Build history of the part. All positions in model axes, mm. Face numbers are marked on the shaded views. A direction names the side the tool comes from. Coordinates: 2 decimals unless noted, no trailing zeros. Loops run counter-clockwise (first coordinate to the right, second up) from the corner with the lowest first, then second, coordinate; pieces in that order, holes last. Notation, with made-up numbers: (81, -2.5) - (93, -2.5) arc R21 ccw to (93, 18.5) - close; hole circle Ø4 at (43.25, 16). An arc over 180 degrees is marked (long way). One line per item, written item: value.
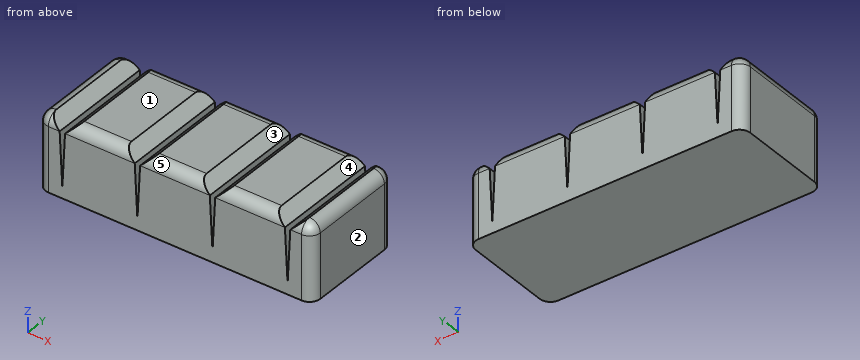
```python
from build123d import *

# Parameters (mm, degrees)
F1_DEPTH = 50
F2_SIZE  = 5
F3_R     = 4.99999


# Not quite as in the source:
# - a fillet or chamfer is up to 0.001 mm smaller than in the source, because OpenCascade refuses the exact size


with BuildPart() as f1:
    # F0 (on Front) → F1 (new body)
    with BuildSketch(Plane.XZ):
        Polygon((-62.637026581, 14.7639395539), (-62.637026581, -20.2360604461), (65.362973419, -20.2360604461), (65.362973419, 14.7639395539), (55.362973419, 14.7639395539), (53.862973419, -15.2360604461), (52.362973419, 14.7639395539), (20.362973419, 14.7639395539), (18.862973419, -15.2360604461), (17.362973419, 14.7639395539), (-14.637026581, 14.7639395539), (-16.137026581, -15.2360604461), (-17.637026581, 14.7639395539), (-49.637026581, 14.7639395539), (-51.137026581, -15.2360604461), (-52.637026581, 14.7639395539), align=None)
    extrude(amount=F1_DEPTH)

    # F2
    f2_edges = [f1.edges().sort_by_distance(p)[0] for p in [
        (-52.637027, -25, 14.76394),
        (-49.637027, -25, 14.76394),
        (-17.637027, -25, 14.76394),
        (-14.637027, -25, 14.76394),
        (17.362973, -25, 14.76394),
        (20.362973, -25, 14.76394),
        (52.362973, -25, 14.76394),
        (55.362973, -25, 14.76394),
    ]]
    chamfer(f2_edges, length=F2_SIZE)

    # F3 (radius 5 in the source; OpenCascade refuses exactly that, so slightly less here)
    f3_edges = [f1.edges().sort_by_distance(p)[0] for p in [
        (-62.637027, -25, 14.76394),
        (-60.137027, -50, 14.76394),
        (-60.137027, 0, 14.76394),
        (-33.637027, -50, 14.76394),
        (-33.637027, 0, 14.76394),
        (1.362973, 0, 14.76394),
        (1.362973, -50, 14.76394),
        (36.362973, -50, 14.76394),
        (36.362973, 0, 14.76394),
        (62.862973, -50, 14.76394),
        (65.362973, -25, 14.76394),
        (62.862973, 0, 14.76394),
        (-62.637027, -50, -2.73606),
        (-62.637027, 0, -2.73606),
        (65.362973, -50, -2.73606),
        (65.362973, 0, -2.73606),
    ]]
    fillet(f3_edges, radius=F3_R)


solid = f1.part
```
Item 1: Probe probe 1 along X at (y, z) = (-39.5, -13); probe 2 along X at (y, z) = (-40, -1.5); probe 3 along Y at (x, z) = (-8, 12). List the from-to ranges inside material, lowest first. Write a range as from..to.
Check result:
probe 1: x = -62.64..-51.25, -51.03..-16.25, -16.03..18.75, 18.97..53.75, 53.97..65.36
probe 2: x = -62.64..-51.82, -50.45..-16.82, -15.45..18.18, 19.55..53.18, 54.55..65.36
probe 3: y = -49.47..-0.53
Item 2: Cut at C-C, the plane z = 4. Write the cut outline in (x, y).
Check result:
outline: (-62.64, -45) arc R5 ccw to (-57.64, -50) - (-52.1, -50) - (-52.1, 0) - (-57.64, 0) arc R5 ccw to (-62.64, -5) - close; (-50.18, -50) - (-17.1, -50) - (-17.1, 0) - (-50.18, 0) - close; (-15.18, -50) - (17.9, -50) - (17.9, 0) - (-15.18, 0) - close; (19.82, -50) - (52.9, -50) - (52.9, 0) - (19.82, 0) - close; (54.82, -50) - (60.36, -50) arc R5 ccw to (65.36, -45) - (65.36, -5) arc R5 ccw to (60.36, 0) - (54.82, 0) - close
Item 3: Cut at A-A, the plane z = -2.5. Write the cut outline in (x, y), then the cut area to 3 significant figures.
Check result:
outline: (-62.64, -45) arc R5 ccw to (-57.64, -50) - (-51.77, -50) - (-51.77, 0) - (-57.64, 0) arc R5 ccw to (-62.64, -5) - close; (-50.5, -50) - (-16.77, -50) - (-16.77, 0) - (-50.5, 0) - close; (-15.5, -50) - (18.23, -50) - (18.23, 0) - (-15.5, 0) - close; (19.5, -50) - (53.23, -50) - (53.23, 0) - (19.5, 0) - close; (54.5, -50) - (60.36, -50) arc R5 ccw to (65.36, -45) - (65.36, -5) arc R5 ccw to (60.36, 0) - (54.5, 0) - close
area: 6,120 mm^2
Item 4: Tool access for the marked faces 4 and 5: list every direction of +Z, -Z, +X, -X, +Y, -Y with a clear straight run to the whole face (end or side of a thin tool).
Check result:
face 4: +Z, +Y, -Y
face 5: +Z, +X, -X, -Y
Item 5: Pull direction X, two halves, no side cores. Call the marked faces 1, 2 and 3: released by +X, released by -X, zero draft, split by the parting line, or undercut.
Check result:
face 1: zero draft
face 2: released by +X
face 3: undercut
Item 6: Cut at D-D, the plane x = -13. Write the cut outline in (y, z).
Check result:
outline: (-50, -20.24) - (0, -20.24) - (0, 9.76) arc R5 ccw to (-0.34, 11.56) - (-49.66, 11.56) arc R5 ccw to (-50, 9.76) - close
